from build123d import *

# Parameters (mm, degrees)
F0_R      = 23.274843
F1_DEPTH  = 25
F2_R      = 26.476855
F3_DEPTH  = 25
F4_R      = 23.196294
F5_DEPTH  = 50
F7_R      = 26.603846
F8_DEPTH  = 40
F9_SIZE   = 5
F11_R     = 26.680042
F12_DEPTH = 40
F13_SIZE  = 5


with BuildPart() as f1:
    # F0 (on Top) → F1 (new body)
    with BuildSketch(Plane.XY):
        Circle(F0_R)
    extrude(amount=F1_DEPTH)

    # F2 (on Top) → F3 (join)
    with BuildSketch(Plane.XY):
        Circle(F2_R)
    extrude(amount=-F3_DEPTH)

    # F4 (on Top) → F5 (join)
    with BuildSketch(Plane.XY):
        Circle(F4_R)
    extrude(amount=-F5_DEPTH)

    # F7 (on offset) → F8 (join)
    with BuildSketch(Plane.XY.offset(-50)):
        Circle(F7_R)
    extrude(amount=-F8_DEPTH)

    # F9
    f9_edges = [f1.edges().sort_by_distance(p)[0] for p in [
        (-26.603846, 0, -90),
    ]]
    chamfer(f9_edges, length=F9_SIZE)

    # F11 (on offset) → F12 (join)
    with BuildSketch(Plane.XY.offset(-90)):
        Circle(F11_R)
    extrude(amount=-F12_DEPTH)

    # F13
    f13_edges = [f1.edges().sort_by_distance(p)[0] for p in [
        (-26.680042, 0, -90),
    ]]
    chamfer(f13_edges, length=F13_SIZE)


solid = f1.part
Work out the finished part from the listing and answer in its coordinate system (mm). A direction names the side the tool comes from. Round coordinates to 2 decimals unless told otherwise and drop trailing zeros. Write each loop counter-clockwise with the first axis right and the second up, starting at its lowest first coordinate (ties: lowest second). Pieces come first, ordered by that corner, then holes. Notation, with made-up numbers: (46, 65) - (71, 65) arc R23 ccw to (71, 83) - close; hole circle Ø9 at (63, 50). An arc over 180 degrees is marked (long way). Answer in a Markdown table with one row per item. Add a question column.
1. The mould has two halves that part along Z. Classify faces 1 (the conical face through (-2.854, 21.736, -90.243)), 2 (the cylindrical face through (-5.784, -26.046, -112.255)), 3 (the flat face through (0, 0, 25)): +Z half, -Z half, draft (parallel to the pull), parting line (faces both ways), or undercut.
2. A cutting plane is placed at A-A, the plane z = -67.5. Determine the outline of the cut face in (x, y).
3. A cutting plane is placed at B-B, the plane y = 0. Determine the outline of the cut face in (x, z), and give its area (3 significant figures).
4. Find the intervals of material crossed by line 1 along Z through (x, y) = (0, 24.5); line 2 along Y through (x, z) = (15.5, -104); line 3 along Z through (x, y) = (22, -6.5), in increasing order. Write a range as from..to.
5. For faces 4 (the conical face through (-4.736, -21.327, -89.757)), 5 (the flat face through (0, 0, -130)), 6 (the flat face through (1.8, -23.4, 0)), determine the directions among +Z, -Z, +X, -X, +Y, -Y from which every point of the face is accessible in a straight line to the end or side of a thin tool.
6. A cutting plane is placed at D-D, the plane z = -107.5. Determine the outline of the cut face in (x, y).
7. Given pin 1 (1.5 mm diameter, centred on y = -14, z = -109.5, fed in from +X); pin 2 (10 mm diameter, centred on y = -9.5, z = -41.5, fed in from -X); pin 3 (1 mm diameter, centred on y = 4, z = -6.5, fed in from -X), each flat-ended and moving along its own axis, determine where each tip first touches the part or whether it passes through.
Worked out:
| question | item | result |
|---|---|---|
| 1 | face 1 | undercut |
| 1 | face 2 | draft |
| 1 | face 3 | +Z half |
| 2 | outline | circle Ø53.21 at (0, 0) |
| 3 | outline | (-26.68, -130) - (26.68, -130) - (26.68, -95) - (21.68, -90) - (21.6, -90) - (26.6, -85) - (26.6, -50) - (23.2, -50) - (23.2, -25) - (26.48, -25) - (26.48, 0) - (23.27, 0) - (23.27, 25) - (-23.27, 25) - (-23.27, 0) - (-26.48, 0) - (-26.48, -25) - (-23.2, -25) - (-23.2, -50) - (-26.6, -50) - (-26.6, -85) - (-21.6, -90) - (-21.68, -90) - (-26.68, -95) - close |
| 3 | area | 7,860 mm^2 |
| 4 | line 1 | -130..-92.82, -87.1..-50, -25..0 |
| 4 | line 2 | -21.72..21.72 |
| 4 | line 3 | -130..-91.26, -88.66..25 |
| 5 | face 4 | none |
| 5 | face 5 | -Z, +X, -X, +Y, -Y |
| 5 | face 6 | +Z |
| 6 | outline | circle Ø53.36 at (0, 0) |
| 7 | pin 1 | x = 23.16 |
| 7 | pin 2 | x = -22.76 |
| 7 | pin 3 | x = -26.24 |
